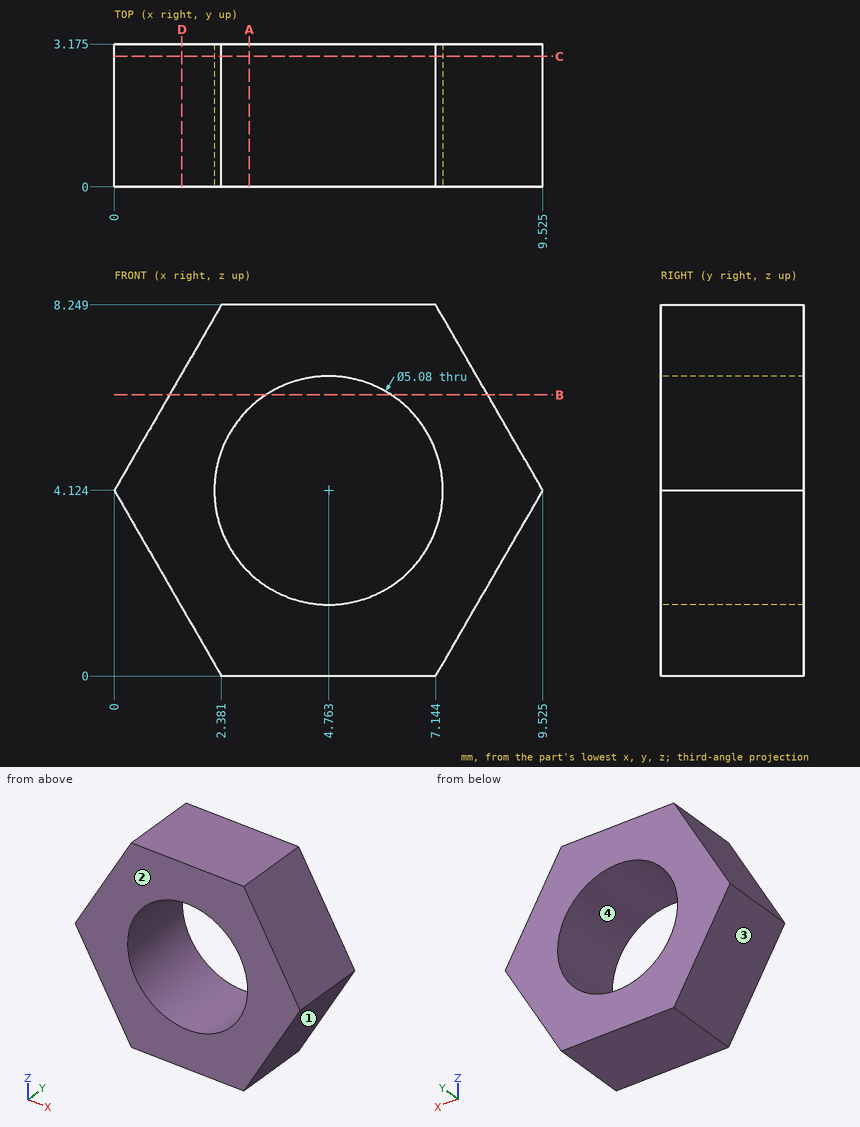
Input: dimensioned drawing with shaded views. Units: mm. Origin: part minimum x, y, z. Give positions to 0.01 mm unless a question says otherwise; leave off trailing zeros. Order: outer loops, then holes, each group sorted by start corner. A loop starts at its lowest first (then second) coordinate and runs counter-clockwise, first axis right, second up. Notation, with made-up numbers: (34, -36.5) -> (43, -36.5) arc R24 ccw to (43, -17.5) -> close; hole circle Ø3 at (34, 82.5). An arc over 180 degrees is marked (long way). Write item = value, one per line.
Item 1: Section query D-D (x = 1.5). Output: boundary loops of the cut face in (y, z) (1 decimal).
Check result:
outline = (0, 1.5) -> (3.2, 1.5) -> (3.2, 6.7) -> (0, 6.7) -> close
Item 2: Section query B-B (z = 6.25). Output: boundary loops of the cut face in (x, y) (1 decimal), then the cut area to 3 significant figures.
Check result:
outline = (1.2, 0) -> (3.4, 0) -> (3.4, 3.2) -> (1.2, 3.2) -> close; (6.2, 0) -> (8.3, 0) -> (8.3, 3.2) -> (6.2, 3.2) -> close
area = 13.6 mm²
Item 3: Ray query, probe 1 along X at (y, z) = (1.9, 2.5) (1 decimal); probe 2 along X at (y, z) = (0.4, 2.75) (1 decimal); probe 3 along Z at (x, y) = (4, 2.5). Return the intervals inside material, ascending.
Check result:
probe_1 = 0.9 to 2.8, 6.7 to 8.6
probe_2 = 0.8 to 2.6, 6.9 to 8.7
probe_3 = 0 to 1.7, 6.55 to 8.25
Item 4: Section query A-A (x = 3). Output: boundary loops of the cut face in (y, z) (1 decimal), then the cut area to 3 significant figures.
Check result:
outline = (0, 0) -> (3.2, 0) -> (3.2, 2.3) -> (0, 2.3) -> close; (0, 6) -> (3.2, 6) -> (3.2, 8.2) -> (0, 8.2) -> close
area = 14.6 mm²
Item 5: Section query C-C (y = 2.9). Output: boundary loops of the cut face in (x, z) (1 decimal).
Check result:
outline = (0, 4.1) -> (2.4, 0) -> (7.1, 0) -> (9.5, 4.1) -> (7.1, 8.2) -> (2.4, 8.2) -> close; hole circle Ø5.1 at (4.8, 4.1)
Item 6: Contact query for flat-ended pins moving along their axis: pin 1 (1 mm diameter, centred on y = 0.5, z = 1.5, fed in from +X); pin 2 (3 mm diameter, centred on x = 4.76, z = 4.12, fed in from +Y); pin 3 (1 mm diameter, centred on x = 8.5, y = 1.5, fed in from -Z) (1 decimal). Output: stop coordinate, or through.
Check result:
pin_1 = 8.3
pin_2 = through
pin_3 = 1.5
Item 7: Mould query, pull axis X, two halves, no side actions, for the marked faces 1, 2, 3 and 4. Classes: +X half, -X half, draft (parallel to the pull), parting line (faces both ways), or undercut.
Check result:
face_1 = +X half
face_2 = draft
face_3 = -X half
face_4 = undercut
